from build123d import *

# Parameters (mm, degrees)
F0_R     = 49.5
F0_R_2   = 1.45
F1_DEPTH = 2.5
F2_R     = 6
F2_R_2   = 1.45
F3_DEPTH = 3.5
F4_R     = 49.5
F5_DEPTH = 15


with BuildPart() as f1:
    # F0 (on Top) → F1 (new body)
    with BuildSketch(Plane.XY):
        Circle(F0_R)
        Circle(F0_R_2, mode=Mode.SUBTRACT)
    extrude(amount=F1_DEPTH)

    # F2 (on face) → F3 (join)
    with BuildSketch(Plane.XY.offset(2.5)):
        Circle(F2_R)
        Circle(F2_R_2, mode=Mode.SUBTRACT)
    extrude(amount=F3_DEPTH)

    # F4 (on face) → F5 (join)
    with BuildSketch(Plane.XY.offset(2.5)):
        Circle(F4_R)
        with BuildLine():
            ThreePointArc((-0.375, 45.875), (31.798359, 32.548359), (45.125, 0.375))
            Line((45.125, 0.375), (48.067823, 2.375))
            ThreePointArc((48.067823, 2.375), (48.106806, 1.375297), (48.125, 0.375))
            ThreePointArc((48.125, 0.375), (34.139349, -33.389349), (0.375, -47.375))
            ThreePointArc((0.375, -47.375), (-32.859019, -33.609019), (-46.625, -0.375))
            ThreePointArc((-46.625, -0.375), (-33.078689, 32.328689), (-0.375, 45.875))
        make_face(mode=Mode.SUBTRACT)
    extrude(amount=F5_DEPTH)


solid = f1.part
Design review of the part built by this model. Coordinates are the model's own, in mm. A direction names the side the tool comes from. Round coordinates to 2 decimals unless told otherwise and drop trailing zeros. Write each loop counter-clockwise with the first axis right and the second up, starting at its lowest first coordinate (ties: lowest second). Pieces come first, ordered by that corner, then holes. Notation, with made-up numbers: (68.5, -9) -> (92.5, -9) arc R21 ccw to (92.5, 12) -> close; hole circle Ø7 at (38, 17.25). An arc over 180 degrees is marked (long way). One line per question, with ' | ' between items.
(1) Draft analysis for pull direction X (two halves, no side actions). For faces 3 (the flat face through (-22, 41, 17.5)), 4 (the flat face through (46.576, 1.361, 9.895)), 5 (the cylindrical face through (-6.44, 49.08, 8.63)), 6 (the cylindrical face through (31.44, 32.9, 9.9)), state which applies: released by +X, released by -X, zero draft, split by the parting line, or undercut.
Result sheet:
face 3: zero draft | face 4: undercut | face 5: split by the parting line | face 6: undercut
(2) Take a section at D-D, the plane x = 4.5. State the section outline as (y, z) points.
Result sheet:
outline: (-49.3, 0) -> (49.3, 0) -> (49.3, 17.5) -> (45.61, 17.5) -> (45.61, 2.5) -> (3.97, 2.5) -> (3.97, 6) -> (-3.97, 6) -> (-3.97, 2.5) -> (-47.2, 2.5) -> (-47.2, 17.5) -> (-49.3, 17.5) -> close
(3) Wall thickness on line 1 (Y direction, x = 0, z = 3.95); line 2 (Z direction, x = 27, y = 13); line 3 (Y direction, x = 0, z = 1.7): over which ranges is each line inside the solid? List them lowest first. Write a range as [from, to].
Result sheet:
line 1: [-49.5, -47.37], [-6, -1.45], [1.45, 6], [45.87, 49.5] | line 2: [0, 2.5] | line 3: [-49.5, -1.45], [1.45, 49.5]
(4) Machinability: for faces 1 (the cylindrical face through (-1.45, 0.06, 2.96)), 2 (the flat face through (1.2, -1.2, 6)), which of the approach directions +Z, -Z, +X, -X, +Y, -Y give a long, thin tool a straight path to every point of the face, cutting with its end or side? Answer none if there is none.
Result sheet:
face 1: +Z, -Z | face 2: +Z
(5) Take a section at A-A, the plane z = 15. State the section outline as (x, y) points (3 decimals), and give its area (3 significant figures).
Result sheet:
outline: circle Ø99 at (0, 0); hole (-46.625, -0.375) arc R47 ccw to (0.375, -47.375) arc R47.75 ccw to (48.125, 0.375) arc R48.127 ccw to (48.068, 2.375) -> (45.125, 0.375) arc R45.5 ccw to (-0.375, 45.875) arc R46.25 ccw to start | area: 862 mm2
(6) Take a section at C-C, the plane x = 23.5. State the section outline as (y, z) points.
Result sheet:
outline: (-43.57, 0) -> (43.57, 0) -> (43.57, 17.5) -> (39.11, 17.5) -> (39.11, 2.5) -> (-41.4, 2.5) -> (-41.4, 17.5) -> (-43.57, 17.5) -> close
(7) Take a section at B-B, the plane y = 38.5. State the section outline as (x, z) points, and give its area (3 significant figures).
Result sheet:
outline: (-31.11, 0) -> (31.11, 0) -> (31.11, 17.5) -> (24.46, 17.5) -> (24.46, 2.5) -> (-25.43, 2.5) -> (-25.43, 17.5) -> (-31.11, 17.5) -> close | area: 341 mm2
(8) Insertion check: P1, Ø5, axis at x = -12.5, z = 10.5, coming from the +Y side; P2, Ø6, axis at y = -34, z = 2, coming from the -X side; P3, Ø1.5, axis at y = -13.5, z = 12.5, coming from the -X side. Each pin has a flat end and moves straight along its axis. Give the tip position at first contact, or say it passes through.
Result sheet:
P1: y = 48.48 | P2: x = -38.59 | P3: x = -47.83
